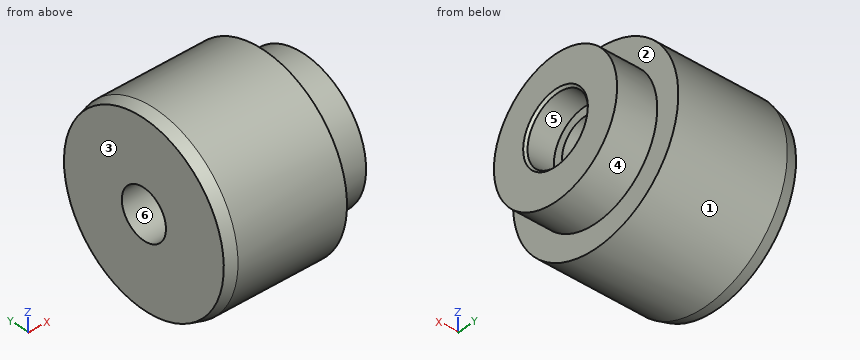
from build123d import *

# Parameters (mm, degrees)
CHAMFER_1_SIZE  = 1
CHAMFER_1_SIZE2 = 0.267949192
CHAMFER_2_SIZE  = 0.2
HOLE_WIZARD_1_D = 4.3


with BuildPart() as part:
    # Эскиз1 → Повернуть1 (revolve)
    with BuildSketch(Plane.XY, mode=Mode.PRIVATE) as revolve_1_sk:
        Polygon((14, 2.95), (11.5, 2.95), (11.5, 0), (0, 0), (0, 8.05), (10.5, 8.05), (10.5, 6), (14, 6), align=None)
    revolve(revolve_1_sk.sketch.rotate(Axis((-5.881924198, 0, 0), (1, 0, 0)), 90), axis=Axis((-5.881924198, 0, 0), (1, 0, 0)))

    # Фаска1
    chamfer_1_edges = [part.edges().sort_by_distance(p)[0] for p in [
        (0, 0, -8.05),
    ]]
    chamfer_1_side = [part.faces().sort_by_distance(p)[0] for p in [
        (5.25, 0, -8.05),
    ]]
    chamfer(chamfer_1_edges, length=CHAMFER_1_SIZE, length2=CHAMFER_1_SIZE2, reference=chamfer_1_side[0])

    # Фаска2
    chamfer_2_edges = [part.edges().sort_by_distance(p)[0] for p in [
        (14, 0, -2.95),
    ]]
    chamfer(chamfer_2_edges, length=CHAMFER_2_SIZE)

    # Отверстие с зазором 1 (through all)
    with Locations(Plane.ZY):
        with Locations((0, 0)):
            Hole(HOLE_WIZARD_1_D / 2)


solid = part.part
Could you check a few things on this model? Use its own coordinates, in mm. Face numbers are marked on the shaded views. A direction names the side the tool comes from. Give positions to 0.01 mm unless a question says otherwise; leave off trailing zeros. Write each loop counter-clockwise with the first axis right and the second up, starting at its lowest first coordinate (ties: lowest second). Pieces come first, ordered by that corner, then holes. Notation, with made-up numbers: (61.5, 71.5) - (94.5, 71.5) arc R13 ccw to (94.5, 93.5) - close; hole circle Ø1 at (5, 40.25). An arc over 180 degrees is marked (long way). Use CSV: the item, a comma, the result in double quotes. Start each with the question number.
Item 1: If I drill on line 1 along Y through (x, z) = (2.5, 0); line 2 along Y through (x, z) = (12.9, 0); line 3 along X through (y, z) = (-2.5, -6.75), over which ranges is the centre line in solid material (lowest first)?
Item 2: I want a section at D-D, the plane x = 6.5. Please give me the cut outline in (y, z).
Item 3: If we mould it in two halves opening along Z, with no side actions, what happens to the marked faces 3, 4, 5 and 6? For each: pulls with the +Z half, pulls with the -Z half, needs draft (parallel to the pull), parting line crosses it, or undercut.
Item 4: For the marked faces 1 and 2, which set-ups out of +Z, -Z, +X, -X, +Y, -Y let a thin tool reach every point of the face, with its end or its side?
Item 5: I'm going to push flat-ended pins straight in: pin 1 (5 mm diameter, centred on x = 3.5, z = -6, fed in from +Y); pin 2 (2 mm diameter, centred on x = 11, y = -4, fed in from -Z); pin 3 (2 mm diameter, centred on x = 4, y = 5, fed in from +Z). Where does each tip first touch, or does it pass through?
Item 6: I want a section at C-C, the plane x = 12. Please give me the cut outline in (y, z), then the cut area to 3 significant figures.
Item 7: I want a section at A-A, the plane z = 0. Please give me the cut outline in (x, y).
Findings:
1,line 1,"y = -8.05 to -2.15, 2.15 to 8.05"
1,line 2,"y = -6 to -2.95, 2.95 to 6"
1,line 3,"x = 0 to 10.5"
2,outline,"circle Ø16.1 at (0, 0); hole circle Ø4.3 at (0, 0)"
3,face 3,"needs draft"
3,face 4,"parting line crosses it"
3,face 5,"undercut"
3,face 6,"undercut"
4,face 1,"+X, -X"
4,face 2,"+X"
5,pin 1,"stops at y = 7.25"
5,pin 2,"stops at z = -7.41"
5,pin 3,"stops at z = 6.99"
6,outline,"circle Ø12 at (0, 0); hole circle Ø5.9 at (0, 0)"
6,area,"85.8 mm2"
7,outline,"(0, -7.78) - (1, -8.05) - (10.5, -8.05) - (10.5, -6) - (14, -6) - (14, -3.15) - (13.8, -2.95) - (11.5, -2.95) - (11.5, -2.15) - (0, -2.15) - close; (0, 2.15) - (11.5, 2.15) - (11.5, 2.95) - (13.8, 2.95) - (14, 3.15) - (14, 6) - (10.5, 6) - (10.5, 8.05) - (1, 8.05) - (0, 7.78) - close"
